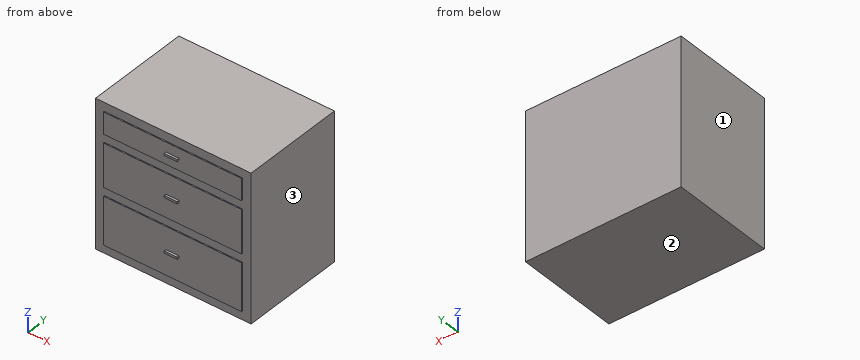
```python
from build123d import *

# Parameters (mm, degrees)
F0_W     = 914.4
F0_H     = 863.6
F1_DEPTH = 609.6
F2_W     = 812.8
F2_H     = 127
F2_H_2   = 254
F2_H_3   = 279.4
F3_DEPTH = 6.35
F4_W     = 76.2
F4_H     = 12.7
F5_DEPTH = 12.7


with BuildPart() as f1:
    # F0 (on Front) → F1 (new body)
    with BuildSketch(Plane.XZ):
        with Locations((-15.939765, 178.42269)):
            Rectangle(F0_W, F0_H)
    extrude(amount=F1_DEPTH)

    # F2 (on face) → F3 (join)
    with BuildSketch(Plane.XZ.offset(609.6)):
        with Locations((-15.939765, 495.92269)):
            Rectangle(F2_W, F2_H)
        with Locations((-15.939765, 254.62269)):
            Rectangle(F2_W, F2_H_2)
        with Locations((-15.939765, -62.87731)):
            Rectangle(F2_W, F2_H_3)
    extrude(amount=F3_DEPTH)

    # F4 (on face) → F5 (join)
    with BuildSketch(Plane.XZ.offset(615.95)):
        with Locations((-15.939765, 495.92269)):
            Rectangle(F4_W, F4_H)
        with Locations((-15.939765, 254.62269)):
            Rectangle(F4_W, F4_H)
        with Locations((-15.939765, -62.87731)):
            Rectangle(F4_W, F4_H)
    extrude(amount=F5_DEPTH)


solid = f1.part
```
Build history of the part. All positions in model axes, mm. Face numbers are marked on the shaded views. Give positions to 0.01 mm unless a question says otherwise; leave off trailing zeros. Order: outer loops, then holes, each group sorted by start corner. A loop starts at its lowest first (then second) coordinate and runs counter-clockwise, first axis right, second up. Notation, with made-up numbers: M 11.5,-27.75 L 58.5,-27.75 A17 ccw 58.5,-7.75 Z; hole C 51,-16 d8. An arc over 180 degrees is marked long. Return JSON: item names as keys, results as strings.
Q1. Band-saw the part on B-B (z = -143). Give the cut face in (x, y), then the cut area to 3 significant figures.
Answer list:
{"outline": "M -473.14,-609.6 L -422.34,-609.6 L -422.34,-615.95 L 390.46,-615.95 L 390.46,-609.6 L 441.26,-609.6 L 441.26,0 L -473.14,0 Z", "area": "563,000 mm^2"}
Q2. Wall check: probe 1 along Y at (x, z) = (-168, 568); probe 2 along Y at (x, z) = (-335, 172.5). Give the ranges that are in metal, low to high. Write a range as from..to.
Answer list:
{"probe 1": "y = -609.6..0", "probe 2": "y = -615.95..0"}
Q3. Flat gauge pins, fed straight in: pin 1 (10 mm diameter, centred on x = -12, y = -621.5, fed in from +Z); pin 2 (6.5 mm diameter, centred on y = -623.5, z = 255.5, fed in from +X); pin 3 (14 mm diameter, centred on x = -0.5, y = -621.5, fed in from +Z). Where does each tip first touch, or does it go through?
Answer list:
{"pin 1": "stops at z = 502.27", "pin 2": "stops at x = 22.16", "pin 3": "stops at z = 559.42"}
Q4. Two-plate mould, pull along X, no slides. Class the marked faces 1, 2 and 3: pulls with the +X half, pulls with the -X half, needs draft (parallel to the pull), parting line crosses it, or undercut.
Answer list:
{"face 1": "pulls with the -X half", "face 2": "needs draft", "face 3": "pulls with the +X half"}
Q5. Band-saw the part on A-A (x = -252). Give the cut face in (y, z), then the cut area to 3 significant figures.
Answer list:
{"outline": "M -615.95,-202.58 L -609.6,-202.58 L -609.6,-253.38 L 0,-253.38 L 0,610.22 L -609.6,610.22 L -609.6,559.42 L -615.95,559.42 L -615.95,432.42 L -609.6,432.42 L -609.6,381.62 L -615.95,381.62 L -615.95,127.62 L -609.6,127.62 L -609.6,76.82 L -615.95,76.82 Z", "area": "531,000 mm^2"}
